```python
from build123d import *

# Parameters (mm, degrees)
F1_DEPTH = 3.175


# Not quite as in the source:
# - a length typed as a fraction of an inch, garbled in the dataset ("3 / 203.2 mm" for 3/8 in), is restored


with BuildPart() as f1:
    # F0 (on Front) → F1 (new body)
    with BuildSketch(Plane.XZ):
        with BuildLine():
            Line((32, -16.05), (35, -16.05))
            Line((35, -16.05), (35, -13.05))
            ThreePointArc((35, -13.05), (33.3469639854, -10.9330653905), (32, -8.6093553766))
            Line((32, -8.6093553766), (32, -16.05))
        make_face()
        with BuildLine():
            ThreePointArc((32, 8.6093553766), (33.3469639854, 10.9330653905), (35, 13.05))
            Line((35, 13.05), (35, 16.05))
            Line((35, 16.05), (32, 16.05))
            Line((32, 16.05), (32, 8.6093553766))
        make_face()
        with BuildLine():
            Line((-35, -16.05), (-32, -16.05))
            Line((-32, -16.05), (-32, -8.6093553766))
            ThreePointArc((-32, -8.6093553766), (-33.3469639854, -10.9330653905), (-35, -13.05))
            Line((-35, -13.05), (-35, -16.05))
        make_face()
        with BuildLine():
            Line((27, -19.05), (32, -19.05))
            Line((32, -19.05), (32, -16.05))
            Line((32, -16.05), (32, -8.6093553766))
            ThreePointArc((32, -8.6093553766), (30.7239047108, -5.268020684), (30.0785620254, -1.75))
            Line((30.0785620254, -1.75), (1.75, -1.75))
            Line((1.75, -1.75), (1.75, -5.45))
            Line((1.75, -5.45), (-1.75, -5.45))
            Line((-1.75, -5.45), (-1.75, -1.75))
            Line((-1.75, -1.75), (-5.5, -1.75))
            Line((-5.5, -1.75), (-5.5, 0))
            Line((-5.5, 0), (-30, 0))
            ThreePointArc((-30, 0), (-30.5065696236, -4.4193042439), (-32, -8.6093553766))
            Line((-32, -8.6093553766), (-32, -16.05))
            Line((-32, -16.05), (-32, -19.05))
            Line((-32, -19.05), (-27, -19.05))
            ThreePointArc((-27, -19.05), (0, -10.05), (27, -19.05))
        make_face()
        with BuildLine():
            ThreePointArc((30.0785620254, 1.75), (30.7239047108, 5.268020684), (32, 8.6093553766))
            Line((32, 8.6093553766), (32, 16.05))
            Line((32, 16.05), (32, 19.05))
            Line((32, 19.05), (27, 19.05))
            ThreePointArc((27, 19.05), (0, 10.05), (-27, 19.05))
            Line((-27, 19.05), (-32, 19.05))
            Line((-32, 19.05), (-32, 16.05))
            Line((-32, 16.05), (-32, 8.6093553766))
            ThreePointArc((-32, 8.6093553766), (-30.5065696236, 4.4193042439), (-30, 0))
            Line((-30, 0), (-5.5, 0))
            Line((-5.5, 0), (-5.5, 1.75))
            Line((-5.5, 1.75), (-1.75, 1.75))
            Line((-1.75, 1.75), (-1.75, 5.45))
            Line((-1.75, 5.45), (1.75, 5.45))
            Line((1.75, 5.45), (1.75, 1.75))
            Line((1.75, 1.75), (30.0785620254, 1.75))
        make_face()
        with BuildLine():
            ThreePointArc((-35, 13.05), (-33.3469639854, 10.9330653905), (-32, 8.6093553766))
            Line((-32, 8.6093553766), (-32, 16.05))
            Line((-32, 16.05), (-35, 16.05))
            Line((-35, 16.05), (-35, 13.05))
        make_face()
    extrude(amount=F1_DEPTH)


solid = f1.part
```
Part model, mm, in its own coordinate system. A direction names the side the tool comes from. Give positions to 0.01 mm unless a question says otherwise; leave off trailing zeros. Loops run counter-clockwise (first coordinate to the right, second up) from the corner with the lowest first, then second, coordinate; pieces in that order, holes last. Notation, with made-up numbers: M 23.25,47 L 41.25,47 A13 ccw 41.25,67 Z; hole C 14.25,26 d7. An arc over 180 degrees is marked long. Return JSON: item names as keys, results as strings.
1) Drill centre lines: line 1 (Z direction, x = 1, y = -1.95); line 2 (X direction, y = -2.85, z = 16); line 3 (Z direction, x = 13.5, y = -1.25). Where is each one in solid material? Low to high.
Calculated:
{"line 1": "z = -10.06 to -5.45, 5.45 to 10.06", "line 2": "x = -35 to -22.36, 22.36 to 35", "line 3": "z = -12.12 to -1.75, 1.75 to 12.12"}
2) Flat gauge pins, fed straight in: pin 1 Ø1 at (y, z) = (-1, -0.5) entering from +X; pin 2 Ø0.9 at (y, z) = (-1, -17.5) entering from +X; pin 3 Ø0.9 at (y, z) = (-1.5, -17) entering from -X. Where does each tip first touch, or does it go through?
Calculated:
{"pin 1": "stops at x = -5.5", "pin 2": "stops at x = 32", "pin 3": "stops at x = -32"}
3) Saw through at B-B, the plane z = -14. List the corners of the cut face in (x, y) (3 decimals).
Calculated:
{"outline": "M -35,-3.175 L -18.436,-3.175 L -18.436,0 L -35,0 Z; M 18.436,-3.175 L 35,-3.175 L 35,0 L 18.436,0 Z"}
4) Saw through at C-C, the plane x = -13. List the corners of the cut face in (y, z) (3 decimals).
Calculated:
{"outline": "M -3.175,-11.969 L 0,-11.969 L 0,11.969 L -3.175,11.969 Z"}
5) Pull direction Z, two halves, no side cores. Call faces 5 (the face through (16, -2, 1.75)), 6 (the face through (32, -2, -18)), 7 (the face through (0, -2, -5.45)), 8 (the face through (0.41, -1.57, 10.05)): released by +Z, released by -Z, zero draft, split by the parting line, or undercut.
Calculated:
{"face 5": "undercut", "face 6": "zero draft", "face 7": "undercut", "face 8": "released by +Z"}
6) Saw through at A-A, the plane x = -3.5. List the corners of the cut face in (y, z) (3 decimals).
Calculated:
{"outline": "M -3.175,-10.186 L 0,-10.186 L 0,-1.75 L -3.175,-1.75 Z; M -3.175,1.75 L 0,1.75 L 0,10.186 L -3.175,10.186 Z"}
7) 3-axis set-ups, long thin cutter, end or side, ignore diameter. For faces 1 (the face through (32, -2, 18)), 2 (the face through (-5.5, -2, 0)), 3 (the face through (-1.75, -2, -4)), 4 (the face through (-32, -2, 18)): which of +Z, -Z, +X, -X, +Y, -Y reach the whole face in a straight line?
Calculated:
{"face 1": "+Z, +X, +Y, -Y", "face 2": "+X, +Y, -Y", "face 3": "+Y, -Y", "face 4": "+Z, -X, +Y, -Y"}
8) Saw through at D-D, the plane z = 7. List the corners of the cut face in (x, y) (3 decimals), then the cut area to 3 significant figures.
Calculated:
{"outline": "M -31.298,-3.175 L 31.298,-3.175 L 31.298,0 L -31.298,0 Z", "area": "199 mm2"}
